The listing builds one solid part. Answer for the finished solid, in the listing's coordinates (mm). A direction names the side the tool comes from. Give positions to 0.01 mm unless a question says otherwise; leave off trailing zeros. Order: outer loops, then holes, each group sorted by start corner. A loop starts at its lowest first (then second) coordinate and runs counter-clockwise, first axis right, second up. Notation, with made-up numbers: (65, 19.5) - (117, 19.5) arc R24 ccw to (117, 32.5) - close; hole circle Ø3 at (-7, 61.25). An arc over 180 degrees is marked (long way). Answer in a Markdown table with one row per item.
from build123d import *

# Parameters (mm, degrees)
CYLINDER004_R          = 7
CYLINDER004_DEPTH      = 1.5
CYLINDER003_R          = 6
CYLINDER003_DEPTH      = 18
FUSION_PLACEMENT_ANGLE = 270


with BuildPart() as cylinder004:
    # Cylinder004 → Cylinder004 (new body)
    with BuildSketch(Plane.XY):
        Circle(CYLINDER004_R)
    extrude(amount=CYLINDER004_DEPTH)


with BuildPart() as dc_jack:
    # Cylinder003 → Cylinder003 (new body)
    with BuildSketch(Plane.XY):
        Circle(CYLINDER003_R)
    extrude(amount=CYLINDER003_DEPTH)

    # Fusion: union Cylinder004
    add(cylinder004.part)


with BuildPart() as dc_jack_1:
    # Fusion placement: moved
    add(dc_jack.part.moved(Location((173.5, -2, 13))).rotate(Axis((173.5, -2, 13), (1, 0, 0)), FUSION_PLACEMENT_ANGLE))


solid = dc_jack_1.part
Item 1: Determine the mould class of faces 3 (the face through (179.966, -1.26, 15.681)), 4 (the face through (173, -2, 13)) for opening direction Z: pulls with the +Z half, pulls with the -Z half, needs draft (parallel to the pull), parting line crosses it, or undercut.
Answer block:
| item | result |
|---|---|
| face 3 | parting line crosses it |
| face 4 | needs draft |
Item 2: Find section B-B on x = 173.5. Write down the section's boundary in (y, z), then the cut area to 3 significant figures.
Answer block:
| item | result |
|---|---|
| outline | (-2, 6) - (-0.5, 6) - (-0.5, 7) - (16, 7) - (16, 19) - (-0.5, 19) - (-0.5, 20) - (-2, 20) - close |
| area | 219 mm² |
Item 3: Find section C-C on y = 6.5. Write down the section's boundary in (x, z).
Answer block:
| item | result |
|---|---|
| outline | circle Ø12 at (173.5, 13) |
Item 4: Find section A-A on z = 13. Write down the section's boundary in (x, y), then the cut area to 3 significant figures.
Answer block:
| item | result |
|---|---|
| outline | (166.5, -2) - (180.5, -2) - (180.5, -0.5) - (179.5, -0.5) - (179.5, 16) - (167.5, 16) - (167.5, -0.5) - (166.5, -0.5) - close |
| area | 219 mm² |
Item 5: Consider line 1 (Y direction, x = 168.5, z = 17.25); line 2 (X direction, y = 4.5, z = 12.75); line 3 (Z direction, x = 169, y = 12.5). Determine where each line is inside the solid, lowest interval first.
Answer block:
| item | result |
|---|---|
| line 1 | -2 to -0.5 |
| line 2 | 167.51 to 179.49 |
| line 3 | 9.03 to 16.97 |
Item 6: Each of these flat-tipped pins is pushed along its axis until it touches: P1, Ø4, axis at x = 172.5, y = 13.5, coming from the -Z side; P2, Ø3, axis at y = 0.5, z = 8.5, coming from the -X side; P3, Ø1.5, axis at x = 172.5, y = 6.5, coming from the +Z side. Where does it stop, or does it pass through?
Answer block:
| item | result |
|---|---|
| P1 | z = 7 |
| P2 | x = 167.37 |
| P3 | z = 18.99 |
Item 7: Which of the six approach directions +Z, -Z, +X, -X, +Y, -Y give full straight-line access (tool end or side, diameter ignored) to faces 1 (the face through (167.506, 7.634, 12.736)), 2 (the face through (173, 16, 13))?
Answer block:
| item | result |
|---|---|
| face 1 | +Y |
| face 2 | +Z, -Z, +X, -X, +Y |
